```python
from build123d import *

# Parameters (mm, degrees)
F0_R     = 1.75
F0_R_2   = 8.05
F0_R_3   = 7
F1_DEPTH = 8
F2_DEPTH = 3.5


with BuildPart() as f1:
    # F0 (on Top) → F1 (new body)
    with BuildSketch(Plane.XY):
        with BuildLine():
            ThreePointArc((-32.905765, 9.292011), (-33.709612, 6.292011), (-35.905765, 4.095859))
            Line((-35.905765, 4.095859), (-14.405765, -33.143234))
            ThreePointArc((-14.405765, -33.143234), (-8.405765, -33.143234), (-5.405765, -38.339386))
            ThreePointArc((-5.405765, -38.339386), (-7.818648, -43.149022), (-13.11663, -44.090294))
            ThreePointArc((-13.11663, -44.090294), (0, -46), (13.116629, -44.090294))
            ThreePointArc((13.116629, -44.090294), (6.596129, -34.752269), (17.405765, -38.339386))
            ThreePointArc((17.405765, -38.339386), (17.20132, -39.8923), (16.601917, -41.339386))
            Line((16.601917, -41.339386), (44.101917, 6.292011))
            ThreePointArc((44.101917, 6.292011), (32.968364, 10.156462), (44.741629, 10.685813))
            ThreePointArc((44.741629, 10.685813), (39.837169, 23), (31.625, 33.404481))
            ThreePointArc((31.625, 33.404481), (33.011352, 31.419083), (33.5, 29.047375))
            ThreePointArc((33.5, 29.047375), (27.5, 23.047375), (21.5, 29.047375))
            Line((21.5, 29.047375), (-21.5, 29.047375))
            ThreePointArc((-21.5, 29.047375), (-29.871708, 23.536023), (-31.625, 33.404481))
            ThreePointArc((-31.625, 33.404481), (-39.837169, 23), (-44.741629, 10.685813))
            ThreePointArc((-44.741629, 10.685813), (-38.204048, 15.250836), (-32.905765, 9.292011))
        make_face()
        with Locations((-8.75, -11.083321)):
            Circle(F0_R, mode=Mode.SUBTRACT)
        with BuildLine():
            ThreePointArc((5, -8.05), (-3.535534, -11.585534), (0, -3.05))
            ThreePointArc((0, -3.05), (3.535534, -4.514466), (5, -8.05))
        make_face(mode=Mode.SUBTRACT)
        with Locations((8.75, -11.083321)):
            Circle(F0_R, mode=Mode.SUBTRACT)
        with Locations((-12, 0)):
            Circle(F0_R_2, mode=Mode.SUBTRACT)
        with BuildLine():
            ThreePointArc((1.75, 4.072124), (1.237437, 2.834687), (0, 2.322124))
            ThreePointArc((0, 2.322124), (-1.237437, 5.309561), (1.75, 4.072124))
        make_face(mode=Mode.SUBTRACT)
        with BuildLine():
            ThreePointArc((20.05, 0), (12, -8.05), (3.95, 0))
            ThreePointArc((3.95, 0), (12, 8.05), (20.05, 0))
        make_face(mode=Mode.SUBTRACT)
        with BuildLine():
            Line((-14.405765, -33.143234), (-35.905765, 4.095859))
            ThreePointArc((-35.905765, 4.095859), (-40.458679, 3.496456), (-44.101917, 6.292011))
            Line((-44.101917, 6.292011), (-16.601917, -41.339386))
            ThreePointArc((-16.601917, -41.339386), (-17.20132, -36.786472), (-14.405765, -33.143234))
        make_face()
        with BuildLine():
            ThreePointArc((-44.101917, 6.292011), (-40.458679, 3.496456), (-35.905765, 4.095859))
            ThreePointArc((-35.905765, 4.095859), (-33.709612, 6.292011), (-32.905765, 9.292011))
            ThreePointArc((-32.905765, 9.292011), (-38.204048, 15.250836), (-44.741629, 10.685813))
            ThreePointArc((-44.741629, 10.685813), (-44.843165, 8.42756), (-44.101917, 6.292011))
        make_face()
        with BuildLine():
            ThreePointArc((-38.030765, 7.776467), (-40.421309, 10.167011), (-37.155765, 9.292011))
            ThreePointArc((-37.155765, 9.292011), (-37.39022, 8.417011), (-38.030765, 7.776467))
        make_face(mode=Mode.SUBTRACT)
        with BuildLine():
            ThreePointArc((-27.5, 35.047375), (-29.720063, 34.62154), (-31.625, 33.404481))
            ThreePointArc((-31.625, 33.404481), (-29.871708, 23.536023), (-21.5, 29.047375))
            ThreePointArc((-21.5, 29.047375), (-23.257359, 33.290016), (-27.5, 35.047375))
        make_face()
        with Locations((-27.5, 29.047375)):
            Circle(F0_R, mode=Mode.SUBTRACT)
        with BuildLine():
            Line((27.5, 35.047375), (-27.5, 35.047375))
            ThreePointArc((-27.5, 35.047375), (-23.257359, 33.290016), (-21.5, 29.047375))
            Line((-21.5, 29.047375), (21.5, 29.047375))
            ThreePointArc((21.5, 29.047375), (23.257359, 33.290016), (27.5, 35.047375))
        make_face()
        with BuildLine():
            ThreePointArc((33.5, 29.047375), (33.011352, 31.419083), (31.625, 33.404481))
            ThreePointArc((31.625, 33.404481), (29.720063, 34.62154), (27.5, 35.047375))
            ThreePointArc((27.5, 35.047375), (23.257359, 33.290016), (21.5, 29.047375))
            ThreePointArc((21.5, 29.047375), (27.5, 23.047375), (33.5, 29.047375))
        make_face()
        with BuildLine():
            ThreePointArc((29.25, 29.047375), (27.5, 27.297375), (25.75, 29.047375))
            ThreePointArc((25.75, 29.047375), (27.5, 30.797375), (29.25, 29.047375))
        make_face(mode=Mode.SUBTRACT)
        with BuildLine():
            ThreePointArc((44.905765, 9.292011), (44.86459, 9.993728), (44.741629, 10.685813))
            ThreePointArc((44.741629, 10.685813), (32.968364, 10.156462), (44.101917, 6.292011))
            ThreePointArc((44.101917, 6.292011), (44.70132, 7.739097), (44.905765, 9.292011))
        make_face()
        with Locations((38.905765, 9.292011)):
            Circle(F0_R, mode=Mode.SUBTRACT)
        with BuildLine():
            ThreePointArc((17.405765, -38.339386), (6.596129, -34.752269), (13.116629, -44.090294))
            ThreePointArc((13.116629, -44.090294), (15.123102, -43.0491), (16.601917, -41.339386))
            ThreePointArc((16.601917, -41.339386), (17.20132, -39.8923), (17.405765, -38.339386))
        make_face()
        with Locations((11.405765, -38.339386)):
            Circle(F0_R, mode=Mode.SUBTRACT)
        with BuildLine():
            ThreePointArc((-5.405765, -38.339386), (-8.405765, -33.143234), (-14.405765, -33.143234))
            ThreePointArc((-14.405765, -33.143234), (-17.20132, -36.786472), (-16.601917, -41.339386))
            ThreePointArc((-16.601917, -41.339386), (-15.123102, -43.0491), (-13.11663, -44.090294))
            ThreePointArc((-13.11663, -44.090294), (-7.818648, -43.149022), (-5.405765, -38.339386))
        make_face()
        with BuildLine():
            ThreePointArc((-9.655765, -38.339386), (-12.280765, -39.854931), (-12.280765, -36.823842))
            ThreePointArc((-12.280765, -36.823842), (-10.530765, -36.823842), (-9.655765, -38.339386))
        make_face(mode=Mode.SUBTRACT)
        with Locations((-12, 0)):
            Circle(F0_R_2)
        with Locations((-12, 0)):
            Circle(F0_R_3, mode=Mode.SUBTRACT)
        with BuildLine():
            ThreePointArc((20.05, 0), (12, 8.05), (3.95, 0))
            ThreePointArc((3.95, 0), (12, -8.05), (20.05, 0))
        make_face()
        with BuildLine():
            ThreePointArc((19, 0), (12, -7), (5, 0))
            ThreePointArc((5, 0), (12, 7), (19, 0))
        make_face(mode=Mode.SUBTRACT)
    extrude(amount=-F1_DEPTH)

    # F0 (on Top) → F2 (cut)
    with BuildSketch(Plane.XY):
        with BuildLine():
            ThreePointArc((20.05, 0), (12, 8.05), (3.95, 0))
            ThreePointArc((3.95, 0), (12, -8.05), (20.05, 0))
        make_face()
        with BuildLine():
            ThreePointArc((19, 0), (12, -7), (5, 0))
            ThreePointArc((5, 0), (12, 7), (19, 0))
        make_face(mode=Mode.SUBTRACT)
        with Locations((-12, 0)):
            Circle(F0_R_2)
        with Locations((-12, 0)):
            Circle(F0_R_3, mode=Mode.SUBTRACT)
    extrude(amount=-F2_DEPTH, mode=Mode.SUBTRACT)


solid = f1.part
```
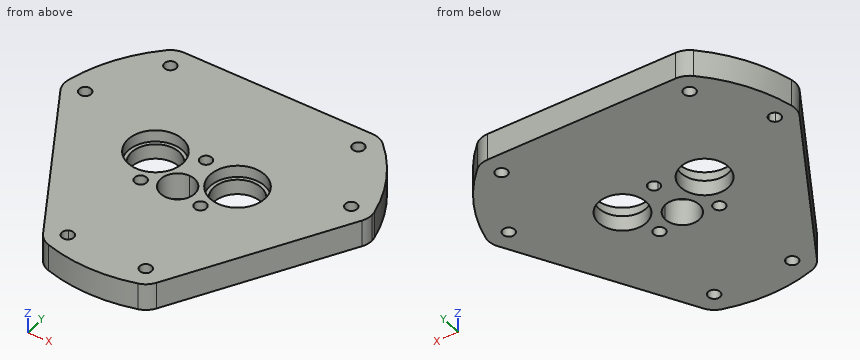
For this review, take the finished solid that the model builds, in its own axes (mm). Coordinates: 2 decimals unless noted, no trailing zeros. Loops run counter-clockwise (first coordinate to the right, second up) from the corner with the lowest first, then second, coordinate; pieces in that order, holes last. Notation, with made-up numbers: (-30, 72.25) -> (24, 72.25) arc R27 ccw to (24, 98.25) -> close; hole circle Ø6 at (-29, 26.5). An arc over 180 degrees is marked (long way). Return JSON: item names as keys, results as strings. Group by question number.
(1) For pin 1 Ø1 at (x, z) = (-4, -6.5) entering from -Y; pin 2 Ø18 at (x, y) = (-12, 0) entering from +Z, all flat-tipped, find the tip position at first contact; note any pin that passes through.
(2) Consider section A-A, the plane x = 12. Give the boundary of the cut face in (y, z), plus the area to 3 significant figures.
(3) Consider section B-B, the plane z = -6.75. Count the separate pieces of the cut face and the enclosed holes in it, plus the area to 3 significant figures.
(4) To check wall thickness, follow L1, parallel to Y at x = 0, z = -2.75; L2, parallel to X at y = 5, z = -5.25; L3, parallel to X at y = 4, z = -5. State the ranges of each line that lie inside material, in increasing order.
(5) Consider section C-C, the plane y = -25. Give the boundary of the cut face in (x, z).
Results below:
{
 "1": {"pin 1": "stops at y = -45.87", "pin 2": "stops at z = 0"},
 "2": {"outline": "(-44.41, -8) -> (-39.99, -8) -> (-39.99, 0) -> (-44.41, 0) -> close; (-36.69, -8) -> (-7, -8) -> (-7, -3.5) -> (-8.05, -3.5) -> (-8.05, 0) -> (-36.69, 0) -> close; (7, -8) -> (35.05, -8) -> (35.05, 0) -> (8.05, 0) -> (8.05, -3.5) -> (7, -3.5) -> close", "area": "490 mm2"},
 "3": {"separate pieces": "1", "enclosed holes": "12", "area": "4,830 mm2"},
 "4": {"L1": "y = -46 to -13.05, -3.05 to 2.32, 5.82 to 35.05", "L2": "x = -43.36 to -16.9, -7.1 to -1.48, 1.48 to 7.1, 16.9 to 43.36", "L3": "x = -42.78 to -17.74, -6.26 to -1.75, 1.75 to 6.26, 17.74 to 42.78"},
 "5": {"outline": "(-26.04, -8) -> (26.04, -8) -> (26.04, 0) -> (-26.04, 0) -> close"}
}
